```python
from build123d import *

# Parameters (mm, degrees)
F2_R     = 5.08
F3_W     = 845.2445566654
F3_H     = 635.8838379383
F4_DEPTH = 25.4


with BuildPart() as f1:
    # F0 (on Front) → F1 (revolve)
    with BuildSketch(Plane.XZ):
        Polygon((-30.6513123214, -11.656133458), (-34.3927890062, 47.0562428236), (-69.5050880313, -29.5000895858), (-30.9391189367, -60.0075013936), (57.4172511697, 3.8853778969), (74.9733969569, -33.8171757758), (124.7637942433, 14.8219969124), (47.3440475762, 25.470810011), align=None)
    revolve(axis=Axis((-51.9489385188, 0, 8.7780766189), (-0.4168899853, 0, -0.9089569518)))

    # F2
    f2_edges = [f1.edges().sort_by_distance(p)[0] for p in [
        (-162.656787, 0, 146.64646),
    ]]
    fillet(f2_edges, radius=F2_R)

    # F3 (on Top) → F4 (join)
    with BuildSketch(Plane.XY):
        with Locations((132.3471516371, -143.5654908419)):
            Rectangle(F3_W, F3_H)
    extrude(amount=F4_DEPTH)


solid = f1.part
```
Check sheet for the modelled part. Datum: model origin and axes. Units: mm. A direction names the side the tool comes from. Give positions to 0.01 mm unless a question says otherwise; leave off trailing zeros. Order: outer loops, then holes, each group sorted by start corner. A loop starts at its lowest first (then second) coordinate and runs counter-clockwise, first axis right, second up. Notation, with made-up numbers: M 42,65 L 58,65 A27 ccw 58,87 Z; hole C 61.25,35 d6. An arc over 180 degrees is marked long. Answer in a Markdown table with one row per item. Add a question column.
Q1. Sectioned sample at A-A, the plane x = -43.5. Count the separate pieces of the cut face and the enclosed holes in it, and give its area (3 significant figures).
Q2. Access from +Z, -Z, +X, -X, +Y, -Y to the whole of each face (thin tool, end or side, straight path). Record for faces 4 (the flat face through (554.969, -148, 13)), 5 (the conical face through (63.697, 1.847, -9.624)), 6 (the flat face through (-20, 1, 25.4)), 7 (the flat face through (-290.275, -148, 13)), 8 (the conical face through (-123.663, -2.397, 49.425)).
Q3. Gauge pin test, flat ends, axial feed: pin 1 Ø3 at (x, y) = (-51, -232) entering from +Z; pin 2 Ø8 at (x, y) = (331, 28) entering from -Z; pin 3 Ø8 at (x, z) = (319, 26) entering from -Y; pin 4 Ø15 at (x, y) = (-22.5, 0.5) entering from -Z. Record the tip position at first contact, or that the pin passes through.
Q4. Thickness scan on L1, parallel to Z at x = -218.5, y = -10; L2, parallel to Z at x = -21, y = 107; L3, parallel to X at y = 64, z = 92. Record the ranges inside material, lowest first.
Q5. Sectioned sample at B-B, the plane y = -170.5. Record the boundary of the cut face in (x, z).
Q6. Sectioned sample at C-C, the plane x = -185.5. Record the boundary of the cut face in (y, z).
Q7. Release check for a two-part mould opening along Y. For faces 1 (the conical face through (-67.22, -0.9, -31.35)), 2 (the flat face through (126, 174.376, 13)), 3 (the conical face through (84.815, 2.26, -24.179)) record: released by +Y, released by -Y, zero draft, split by the parting line, or undercut.
Verdict:
| question | item | result |
|---|---|---|
| 1 | separate pieces | 1 |
| 1 | enclosed holes | 4 |
| 1 | area | 29,200 mm² |
| 2 | face 4 | +Z, -Z, +X, +Y, -Y |
| 2 | face 5 | -Z |
| 2 | face 6 | +Z |
| 2 | face 7 | +Z, -Z, -X, +Y, -Y |
| 2 | face 8 | none |
| 3 | pin 1 | z = 25.4 |
| 3 | pin 2 | z = 0 |
| 3 | pin 3 | y = -461.51 |
| 3 | pin 4 | z = -59.33 |
| 4 | L1 | 0 to 25.4 |
| 4 | L2 | 0 to 25.4, 33.26 to 64.73 |
| 4 | L3 | -151.71 to -89.81 |
| 5 | outline | M -290.28,0 L 554.97,0 L 554.97,25.4 L -290.28,25.4 Z |
| 6 | outline | M -461.51,0 L 174.38,0 L 174.38,25.4 L -461.51,25.4 Z |
| 7 | face 1 | undercut |
| 7 | face 2 | released by +Y |
| 7 | face 3 | split by the parting line |
